Verification items for the finished model (mm, model axes). Give positions to 0.01 mm unless a question says otherwise; leave off trailing zeros. Order: outer loops, then holes, each group sorted by start corner. A loop starts at its lowest first (then second) coordinate and runs counter-clockwise, first axis right, second up.
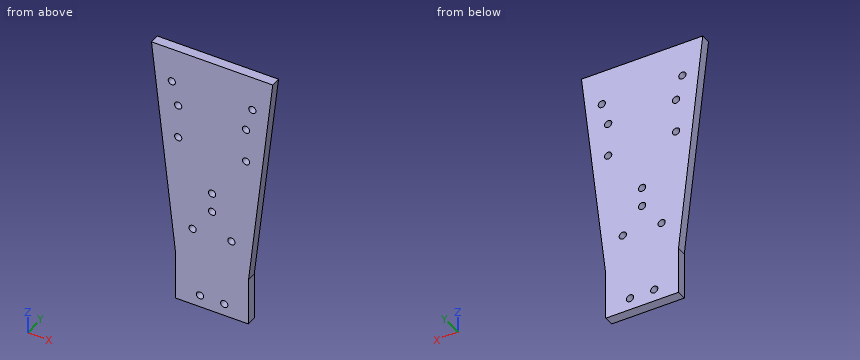
from build123d import *

# Parameters (mm, degrees)
EXTRUDE_1_DEPTH     = 4
SKETCH_4_R          = 1.5
CUT_EXTRUDE_3_DEPTH = 99.569772243
SKETCH_5_R          = 1.5
CUT_EXTRUDE_4_DEPTH = 99.569772243
SKETCH_9_R          = 1.5
CUT_EXTRUDE_6_DEPTH = 10
SKETCH_10_W         = 30
SKETCH_10_H         = 4
EXTRUDE_2_DEPTH     = 19.5
SKETCH_11_R         = 1.5
CUT_EXTRUDE_7_DEPTH = 99.569772243


with BuildPart() as part:
    # 草图1 → 凸台-拉伸1 (new body)
    with BuildSketch(Plane(origin=(0, 0, 0), x_dir=(1, 0, 0), z_dir=(0, 1, 0))):
        Polygon((0, 0), (30, 0), (40, -90), (-10, -90), align=None)
    extrude(amount=EXTRUDE_1_DEPTH)

    # 草图4 → 切除-拉伸3 (cut, through all)
    with BuildSketch(Plane(origin=(0, 4, 0), x_dir=(1, 0, 0), z_dir=(0, 1, 0))):
        with Locations(Location((1, -66, 0), (0, 0, 270))):
            Circle(SKETCH_4_R)
        with Locations(Location((1, -52, 0), (0, 0, 270))):
            Circle(SKETCH_4_R)
        with Locations(Location((29, -66, 0), (0, 0, 270))):
            Circle(SKETCH_4_R)
        with Locations(Location((29, -52, 0), (0, 0, 270))):
            Circle(SKETCH_4_R)
    extrude(amount=-CUT_EXTRUDE_3_DEPTH, mode=Mode.SUBTRACT)

    # 草图5 → 切除-拉伸4 (cut, through all)
    with BuildSketch(Plane(origin=(0, 4, 0), x_dir=(1, 0, 0), z_dir=(0, 1, 0))):
        with Locations(Location((15, -32.4, 0), (0, 0, 270))):
            Circle(SKETCH_5_R)
        with Locations(Location((15, -24.4, 0), (0, 0, 270))):
            Circle(SKETCH_5_R)
    extrude(amount=-CUT_EXTRUDE_4_DEPTH, mode=Mode.SUBTRACT)

    # 草图9 → 切除-拉伸6 (cut)
    with BuildSketch(Plane(origin=(0, 4, 0), x_dir=(1, 0, 0), z_dir=(0, 1, 0))):
        with Locations(Location((6.963154721, -13.77878744, 0), (0, 0, 270))):
            Circle(SKETCH_9_R)
        with Locations(Location((22.953054881, -14.34720003, 0), (0, 0, 270))):
            Circle(SKETCH_9_R)
        with Locations(Location((-1.6, -75.75, 0), (0, 0, 270))):
            Circle(SKETCH_9_R)
        with Locations(Location((31.6, -75.75, 0), (0, 0, 270))):
            Circle(SKETCH_9_R)
    extrude(amount=-CUT_EXTRUDE_6_DEPTH, mode=Mode.SUBTRACT)

    # 草图10 → 凸台-拉伸2 (add)
    with BuildSketch(Plane(origin=(0, 0, 0), x_dir=(-1, 0, 0), z_dir=(0, 0, -1))):
        with Locations((-15, 2)):
            Rectangle(SKETCH_10_W, SKETCH_10_H)
    extrude(amount=EXTRUDE_2_DEPTH)

    # 草图11 → 切除-拉伸7 (cut, through all)
    with BuildSketch(Plane.XZ):
        with Locations(Location((10, -14.5, 0), (0, 0, 270))):
            Circle(SKETCH_11_R)
        with Locations(Location((20, -14.5, 0), (0, 0, 270))):
            Circle(SKETCH_11_R)
    extrude(amount=-CUT_EXTRUDE_7_DEPTH, mode=Mode.SUBTRACT)


solid = part.part
(1) Section check A-A, the plane x = 31.6. Enter the section's corners in (y, z).
Solved:
outline: (0, 14.4) - (4, 14.4) - (4, 74.25) - (0, 74.25) - close; (0, 77.25) - (4, 77.25) - (4, 90) - (0, 90) - close
(2) Go/stop test with flat-tipped pins: pin 1 (2.5 mm diameter, centred on x = 29, z = 52, fed in from -Y); pin 2 (1 mm diameter, centred on y = 2, z = 60.5, fed in from -X). Record where each tip stops, or that it passes through.
Solved:
pin 1: passes through
pin 2: stops at x = -6.78
(3) Section check C-C, the plane x = 1. Enter the section's corners in (y, z), then the cut area to 3 significant figures.
Solved:
outline: (0, -19.5) - (4, -19.5) - (4, 50.5) - (0, 50.5) - close; (0, 53.5) - (4, 53.5) - (4, 64.5) - (0, 64.5) - close; (0, 67.5) - (4, 67.5) - (4, 90) - (0, 90) - close
area: 414 mm2
(4) Scan lines: line 1 (X direction, y = 3.1, z = 52); line 2 (X direction, y = 2, z = 65); line 3 (Z direction, x = 14.5, y = 2.6). Record each from-to range of solid material in increasing order.
Solved:
line 1: x = -5.78 to -0.5, 2.5 to 27.5, 30.5 to 35.78
line 2: x = -7.22 to -0.12, 2.12 to 27.88, 30.12 to 37.22
line 3: z = -19.5 to 22.99, 25.81 to 30.99, 33.81 to 90
(5) Section check B-B, the plane z = 75.75. Enter the section's corners in (x, y).
Solved:
outline: (-8.42, 0) - (-3.1, 0) - (-3.1, 4) - (-8.42, 4) - close; (-0.1, 0) - (30.1, 0) - (30.1, 4) - (-0.1, 4) - close; (33.1, 0) - (38.42, 0) - (38.42, 4) - (33.1, 4) - close
(6) Section check D-D, the plane y = 0.9. Give the number of separate pieces and of enclosed holes in the cut face, then the cut area to 3 significant figures.
Solved:
separate pieces: 1
enclosed holes: 12
area: 4,100 mm2
